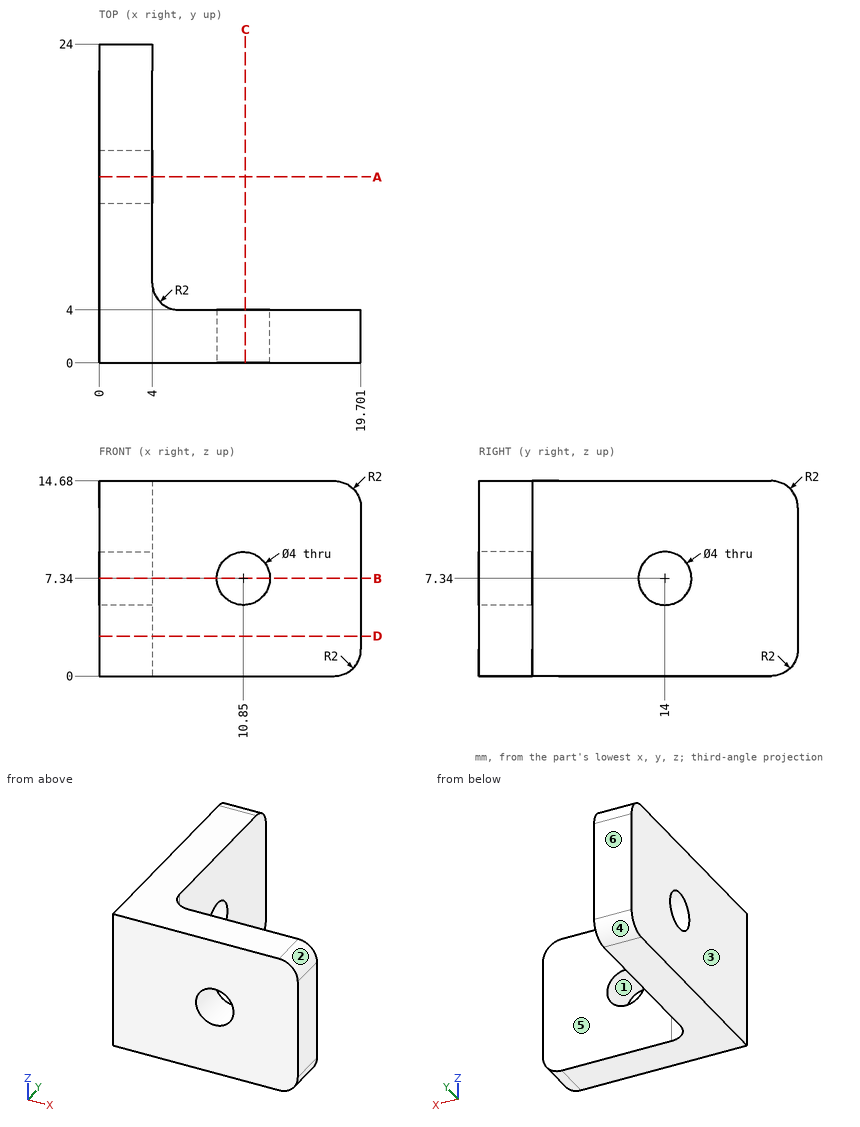
Here's the drawing with two shaded views (mm, measured from the low corner). I have some questions. A direction names the side the tool comes from. Round coordinates to 2 decimals unless told otherwise and drop trailing zeros. Loops run counter-clockwise (first coordinate to the right, second up) from the corner with the lowest first, then second, coordinate; pieces in that order, holes last. Notation, with made-up numbers: (29.5, 29.25) -> (69.5, 29.25) arc R24 cw to (69.5, 54.25) -> close; hole circle Ø4 at (54, -36). An arc over 180 degrees is marked (long way). Answer as CSV lines item,"result". Start each with the question number.
1. I'm going to push flat-ended pins straight in: P1, Ø4, axis at x = 12.5, z = 9.5, coming from the +Y side; P2, Ø3, axis at y = 14, z = 7.34, coming from the +X side. Where does each tip first touch, or does it pass through?
2. I need wall thicknesses on probe 1 along Y at (x, z) = (0.95, 7.34); probe 2 along X at (y, z) = (2.1, 7.34); probe 3 along X at (y, z) = (11.25, 4). Which ranges of each line are inside material? Lowest first, please. Write a range as from..to.
3. Imagine slicing it at A-A on y = 14. Write out the boundary of the cut face in (x, z), plus the area to 3 significant figures.
4. Imagine slicing it at C-C on x = 11. Write out the boundary of the cut face in (y, z) (1 decimal).
5. For the marked faces 5 and 6, which set-ups out of +Z, -Z, +X, -X, +Y, -Y let a thin tool reach every point of the face, with its end or its side?
6. Imagine slicing it at D-D on z = 3. Write out the boundary of the cut face in (x, y).
7. If we mould it in two halves opening along Z, with no side actions, what happens to the marked faces 1, 2, 3 and 4? For each: pulls with the +Z half, pulls with the -Z half, needs draft (parallel to the pull), parting line crosses it, or undercut.
8. Imagine slicing it at B-B on z = 7.34. Write out the boundary of the cut face in (x, y).
Solution:
1,P1,"y = 4"
1,P2,"through"
2,probe 1,"0..12, 16..24"
2,probe 2,"0..8.85, 12.85..19.7"
2,probe 3,"0..4"
3,outline,"(0, 0) -> (4, 0) -> (4, 5.34) -> (0, 5.34) -> close; (0, 9.34) -> (4, 9.34) -> (4, 14.68) -> (0, 14.68) -> close"
3,area,"42.7 mm²"
4,outline,"(0, 0) -> (4, 0) -> (4, 5.3) -> (0, 5.3) -> close; (0, 9.3) -> (4, 9.3) -> (4, 14.7) -> (0, 14.7) -> close"
5,face 5,"+Z, -Z, +X, +Y"
5,face 6,"+Z, -Z, +X, -X, +Y"
6,outline,"(0, 0) -> (19.7, 0) -> (19.7, 4) -> (6, 4) arc R2 cw to (4, 6) -> (4, 24) -> (0, 24) -> close"
7,face 1,"undercut"
7,face 2,"pulls with the +Z half"
7,face 3,"needs draft"
7,face 4,"pulls with the -Z half"
8,outline,"(0, 0) -> (8.85, 0) -> (8.85, 4) -> (6, 4) arc R2 cw to (4, 6) -> (4, 12) -> (0, 12) -> close; (0, 16) -> (4, 16) -> (4, 24) -> (0, 24) -> close; (12.85, 0) -> (19.7, 0) -> (19.7, 4) -> (12.85, 4) -> close"
